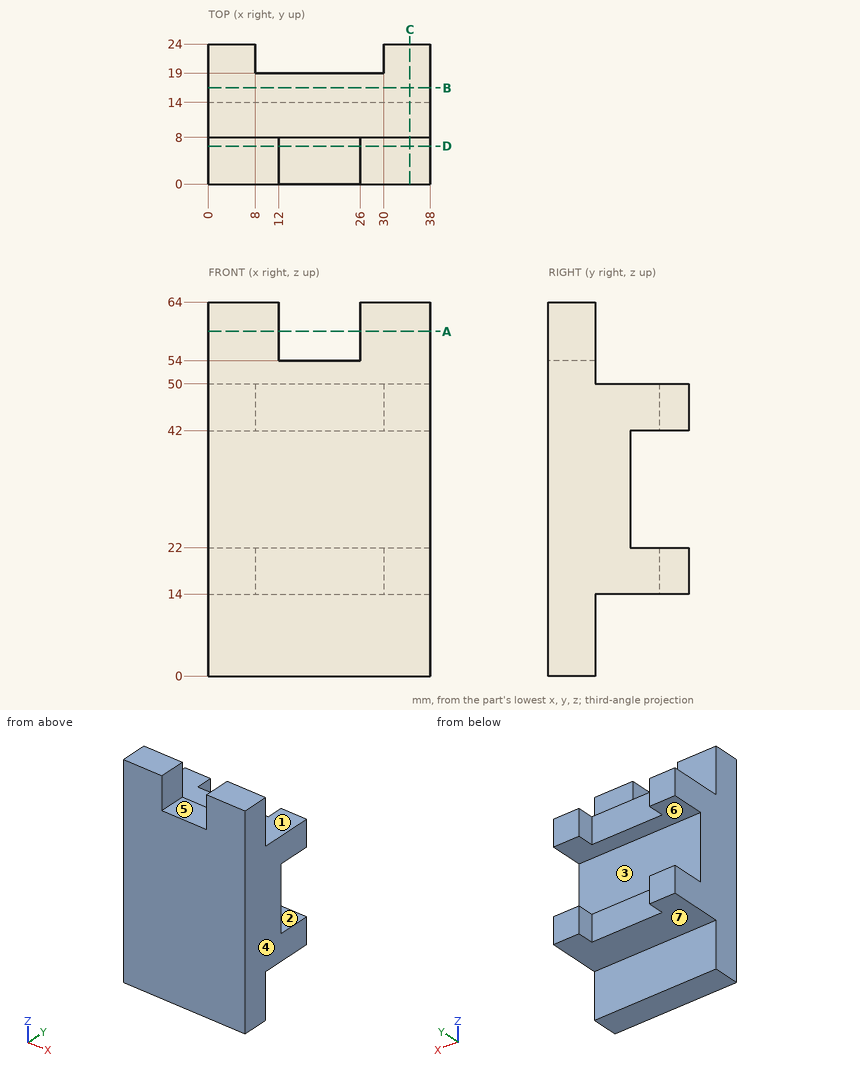
Input: dimensioned drawing with shaded views. Units: mm. Origin: part minimum x, y, z. A direction names the side the tool comes from. Round coordinates to 2 decimals unless told otherwise and drop trailing zeros. Order: outer loops, then holes, each group sorted by start corner. A loop starts at its lowest first (then second) coordinate and runs counter-clockwise, first axis right, second up.
Q1. Mould query, pull axis Z, two halves, no side actions, for the marked faces 1, 2, 3 and 4. Classes: released by +Z, released by -Z, zero draft, split by the parting line, or undercut.
Result sheet:
face 1: released by +Z
face 2: undercut
face 3: undercut
face 4: zero draft
Q2. Section D-D, the plane y = 6.5. Output: boundary loops of the cut face in (x, z), and give its area (3 significant figures).
Result sheet:
outline: (0, 0) - (38, 0) - (38, 64) - (26, 64) - (26, 54) - (12, 54) - (12, 64) - (0, 64) - close
area: 2,290 mm2
Q3. Section C-C, the plane x = 34.5. Output: boundary loops of the cut face in (y, z), and give its area (3 significant figures).
Result sheet:
outline: (0, 0) - (8, 0) - (8, 14) - (24, 14) - (24, 22) - (14, 22) - (14, 42) - (24, 42) - (24, 50) - (8, 50) - (8, 64) - (0, 64) - close
area: 888 mm2
Q4. Section A-A, the plane z = 59. Output: boundary loops of the cut face in (x, y).
Result sheet:
outline: (0, 0) - (12, 0) - (12, 8) - (0, 8) - close; (26, 0) - (38, 0) - (38, 8) - (26, 8) - close
Q5. Section B-B, the plane y = 16.5. Output: boundary loops of the cut face in (x, z), and give its area (3 significant figures).
Result sheet:
outline: (0, 14) - (38, 14) - (38, 22) - (0, 22) - close; (0, 42) - (38, 42) - (38, 50) - (0, 50) - close
area: 608 mm2
Q6. Access query for the marked faces 5, 6 and 7. Directions: +Z, -Z, +X, -X, +Y, -Y. A direction counts if a zero-diameter tool reaches every point of the face in a straight line with its end or side. Return the directions, or none.
Result sheet:
face 5: +Z, +Y, -Y
face 6: +X, -X, +Y
face 7: -Z, +X, -X, +Y
Q7. Pin query (flat end, axial travel): pin 1 (2 mm diameter, centred on x = 28.5, y = 2.5, fed in from -Z); pin 2 (1 mm diameter, centred on y = 18, z = 24, fed in from -X); pin 3 (3 mm diameter, centred on x = 19.5, y = 19.5, fed in from +Z); pin 4 (6.5 mm diameter, centred on x = 22, z = 45, fed in from +Y). Return the tip coordinate at first contact, or that it passes through.
Result sheet:
pin 1: stops at z = 0
pin 2: passes through
pin 3: stops at z = 50
pin 4: stops at y = 19
Q8. Material intervals for probe 1 along Z at (x, y) = (34.5, 16.75); probe 2 along Y at (x, z) = (28, 58); probe 3 along Y at (x, z) = (6.5, 30), sorted ascending.
Result sheet:
probe 1: z = 14 to 22, 42 to 50
probe 2: y = 0 to 8
probe 3: y = 0 to 14
